Geometry: final body of the model. Coordinates: model frame, mm. A direction names the side the tool comes from. Round coordinates to 2 decimals unless told otherwise and drop trailing zeros. Loops run counter-clockwise (first coordinate to the right, second up) from the corner with the lowest first, then second, coordinate; pieces in that order, holes last. Notation, with made-up numbers: M -30.75,71.5 L 3.25,71.5 A20 ccw 3.25,89.5 Z; hole C 35.5,-1 d3. An arc over 180 degrees is marked long. Return JSON: item names as keys, results as strings.
Autodesk Fusion 360 part; units mm, degrees
sketch "Sketch1" plane through (0, 0, 0) normal (0, 0, 1) x (1, 0, 0)
  line L0 (0, 0) -> (18, 0)
  line L1 (18, 0) -> (18, -18)
  line L2 (18, -18) -> (0, -18)
  line L3 (0, -18) -> (0, 0)
  line L4 (11.5, -10.3) -> (6.5, -10.3)
  line L5 (6.5, -10.3) -> (6.5, -7.7)
  line L6 (6.5, -7.7) -> (11.5, -7.7)
  line L7 (11.5, -7.7) -> (11.5, -10.3)
  line L8 (11.5, -10.3) -> (6.5, -7.7) construction
  line L9 (6.5, -10.3) -> (11.5, -7.7) construction
  line L10 (11.1, -9.6) -> (6.9, -9.6)
  line L11 (6.9, -9.6) -> (6.9, -8.4)
  line L12 (6.9, -8.4) -> (11.1, -8.4)
  line L13 (11.1, -8.4) -> (11.1, -9.6)
  line L14 (11.1, -9.6) -> (6.9, -8.4) construction
  line L15 (6.9, -9.6) -> (11.1, -8.4) construction
  line L16 (7.7, -6.5) -> (10.3, -11.5) construction
  line L17 (8.4, -11.1) -> (9.6, -6.9) construction
  line L18 (7.7, -11.5) -> (10.3, -6.5) construction
  line L19 (7.7, -6.5) -> (10.3, -6.5)
  line L20 (8.4, -11.1) -> (8.4, -6.9)
  line L21 (7.7, -11.5) -> (7.7, -6.5)
  line L22 (8.4, -6.9) -> (9.6, -11.1) construction
  line L23 (10.3, -6.5) -> (10.3, -11.5)
  line L24 (10.3, -11.5) -> (7.7, -11.5)
  line L25 (9.6, -6.9) -> (9.6, -11.1)
  line L26 (9.6, -11.1) -> (8.4, -11.1)
  line L27 (8.4, -6.9) -> (9.6, -6.9)
  line L28 (17.3, -0.7) -> (0.7, -0.7)
  line L29 (0.7, -0.7) -> (0.7, -17.3)
  line L30 (0.7, -17.3) -> (17.3, -17.3)
  line L31 (17.3, -17.3) -> (17.3, -0.7)
  line L32 (17.3, -0.7) -> (0.7, -17.3) construction
  line L33 (0.7, -0.7) -> (17.3, -17.3) construction
  point P0 (9, -9)
  point P1 (9, -9)
  point P2 (9, -9)
  point P3 (9, -9)
  point P4 (9, -9)
  dimension "d1" = 18
  dimension "d2" = 18
  dimension "d9" = 5
  dimension "d10" = 2.6
  dimension "d11" = 4.2
  dimension "d12" = 1.2
  dimension "d13" = 5
  dimension "d14" = 2.6
  dimension "d15" = 4.2
  dimension "d16" = 1.2
  dimension "d21" = 16.6
  dimension "d22" = 16.6
extrude "Extrude1" add sketch "Sketch1" along normal blind 4.9 contours L0 L1 L2 L3 | L4 L6 L7 L10 L12 L13 L23 | L4 L20 L21 L23 L24 L25 L26 | L4 L10 L23 L25 | L4 L20 L25 L26 | L4 L10 L20 L25 | L10 L12 L13 L23 | L10 L12 L23 L25 | L6 L12 L23 L25 | L6 L19 L20 L21 L23 L25 L27 | L4 L10 L20 L21 | L10 L12 L20 L25 | L6 L12 L20 L25 | L6 L20 L25 L27 | L4 L5 L6 L10 L11 L12 L21 | L10 L12 L20 L21 | L6 L12 L20 L21 | L10 L11 L12 L21 | L28 L29 L30 L31
fillet "Fillet1" radius 2 4 edges at (18, -18, 2.45) (18, 0, 2.45) (0, 0, 2.45) (0, -18, 2.45)
extrude "Extrude2" cut sketch "Sketch1" along normal blind 3.4 contours L4 L6 L7 L10 L12 L13 L23 | L4 L20 L21 L23 L24 L25 L26 | L4 L10 L23 L25 | L4 L20 L25 L26 | L4 L10 L20 L25 | L10 L12 L13 L23 | L10 L12 L23 L25 | L6 L12 L23 L25 | L6 L19 L20 L21 L23 L25 L27 | L4 L10 L20 L21 | L10 L12 L20 L25 | L6 L12 L20 L25 | L6 L20 L25 L27 | L4 L5 L6 L10 L11 L12 L21 | L10 L12 L20 L21 | L6 L12 L20 L21 | L10 L11 L12 L21 | L28 L29 L30 L31
fillet "Fillet2" radius 1.3 4 edges at (17.3, -17.3, 1.7) (0.7, -17.3, 1.7) (0.7, -0.7, 1.7) (17.3, -0.7, 1.7)
extrude "Extrude3" add sketch "Sketch1" along normal blind 5 from surface at -1 contours L4 L6 L7 L10 L12 L13 L23 | L4 L20 L21 L23 L24 L25 L26 | L4 L10 L23 L25 | L6 L12 L23 L25 | L6 L19 L20 L21 L23 L25 L27 | L4 L10 L20 L21 | L4 L5 L6 L10 L11 L12 L21 | L6 L12 L20 L21
fillet "Fillet3" radius 0.5 8 edges at (10.3, -11.5, 1.2) (11.5, -10.3, 1.2) (11.5, -7.7, 1.2) (10.3, -6.5, 1.2) (7.7, -6.5, 1.2) (6.5, -7.7, 1.2) (6.5, -10.3, 1.2) (7.7, -11.5, 1.2)
ref_plane "WorkPlane1" through (0, 0, 36.4) normal (0, 0, 1) x (1, 0, 0)
sketch "Sketch2" plane through (0, 0, 36.4) normal (0, 0, 1) x (1, 0, 0)
  point P0 (9, -9)
sphere "SpherePrimitive1" cut diameter 65 placed x (1, 0, 0) y (0, 1, 0) z (0, 0, 1) at (9, -9, 36.4)
fillet "Fillet4" radius 1 8 edges at (17.4142, -17.4142, 4.9) (18, -9, 4.9) (17.4142, -0.5858, 4.9) (9, 0, 4.9) (0.5858, -0.5858, 4.9) (0, -9, 4.9) (0.5858, -17.4142, 4.9) (9, -18, 4.9)
equation "d21 = 18 mm - 1.4 mm"
equation "d22 = 18 mm - 1.4 mm"
equation "d23 = 4.9 mm - ( 4.9 mm - 3.4 mm )"
equation "d32 = 31.5 mm + 4.9 mm"
Q1. Pull-direction query (Y, two-part tool) for faces 1 (the flat face through (0.7, -9, 2)), 2 (the cylindrical face through (17.4, -17.43, 1.98)), 3 (the cylindrical face through (17.43, -0.6, 1.98)), 4 (the flat face through (9.6, -8, 1)); classes: pulls with the +Y half, pulls with the -Y half, needs draft (parallel to the pull), parting line crosses it, or undercut.
Determined:
{"face 1": "undercut", "face 2": "pulls with the -Y half", "face 3": "pulls with the +Y half", "face 4": "undercut"}
Q2. Section query C-C (x = 14.75). Output: boundary loops of the cut face in (y, z).
Determined:
{"outline": "M -18,0 L -17.3,0 L -17.3,3.4 L -0.7,3.4 L -0.7,0 L 0,0 L 0,3.9 A1 ccw -1,4.9 L -3.44,4.9 A31.99 cw -14.56,4.9 L -17,4.9 A1 ccw -18,3.9 Z"}
Q3. Section query B-B (z = 2.9). State how many separate pieces and enclosed holes the cut face has, plus the area to 3 significant figures.
Determined:
{"separate pieces": "2", "enclosed holes": "2", "area": "56.6 mm^2"}
Q4. Material intervals for L1, parallel to X at y = -10.75, z = 0.05; L2, parallel to X at y = -3, z = 2.8; L3, parallel to X at y = -10, z = 0.6, sorted ascending.
Determined:
{"L1": "x = 0 to 0.7, 7.7 to 8.4, 9.6 to 10.3, 17.3 to 18", "L2": "x = 0 to 0.7, 17.3 to 18", "L3": "x = 0 to 0.7, 6.54 to 8.4, 9.6 to 11.46, 17.3 to 18"}
Q5. Pin query (flat end, axial travel): pin 1 (4 mm diameter, centred on x = 10.5, y = -7, fed in from +Z); pin 2 (3 mm diameter, centred on x = 7.5, y = -11, fed in from +Z). Return the tip coordinate at first contact, or that it passes through.
Determined:
{"pin 1": "stops at z = 4.21", "pin 2": "stops at z = 4.15"}
Q6. Section query D-D (y = -14.5). Output: boundary loops of the cut face in (x, z).
Determined:
{"outline": "M 0,0 L 0.7,0 L 0.7,3.4 L 17.3,3.4 L 17.3,0 L 18,0 L 18,3.9 A1 ccw 17,4.9 L 14.81,4.9 A32.03 cw 3.19,4.9 L 1,4.9 A1 ccw 0,3.9 Z"}
Q7. Reachability of faces 5 (the cylindrical face through (16.91, -16.93, 1.72)), 6 (the cylindrical face through (8.902, -17.715, 4.599)) from +Z, -Z, +X, -X, +Y, -Y: full face, straight path, thin tool, end or side. Return the list, or none.
Determined:
{"face 5": "-Z", "face 6": "+Z, +X, -X, -Y"}
